CAD build for the part. Positions are in the model's coordinates, mm. A direction names the side the tool comes from. Round coordinates to 2 decimals unless told otherwise and drop trailing zeros. Write each loop counter-clockwise with the first axis right and the second up, starting at its lowest first coordinate (ties: lowest second). Pieces come first, ordered by that corner, then holes. Notation, with made-up numbers: (48.25, 67) - (73.25, 67) arc R38 ccw to (73.25, 105) - close; hole circle Ø8 at (-18.5, 49). An arc over 180 degrees is marked (long way). Use one line per item in the form item = value. Start each with the question number.
Item 1: Pull direction Y, two halves, no side cores. Call faces 4 (the conical face through (-1.429, -3.625, 10.887)), 5 (the flat face through (-1.968, 11, 0)), 6 (the flat face through (0, 6.35, 5)): +Y half, -Y half, draft (parallel to the pull), parting line (faces both ways), or undercut.
Item 2: Tool access for faces 1 (the cylindrical face through (21.804, 3.131, -6.867)), 2 (the flat face through (0, 0, 15)), 3 (the flat face through (1.968, 11, 0)): list every direction of +Z, -Z, +X, -X, +Y, -Y with a clear straight run to the whole face (end or side of a thin tool).
Item 3: Band-saw the part on A-A, the plane y = -183.5. List the corners of the cut face in (x, z) (3 decimals).
Item 4: Pin check, flat tips, straight feed: pin 1 (1 mm diameter, centred on x = -7, y = -152.5, fed in from -Z); pin 2 (5 mm diameter, centred on x = -18, z = 0, fed in from +Y); pin 3 (2.5 mm diameter, centred on y = 10, z = 0.5, fed in from -X). Stop position of each tip, or through.
Item 5: Drill centre lines: L1, parallel to X at y = 4, z = 0; L2, parallel to Z at x = -1, y = -251. Where is each one in solid material? Low to high.
from build123d import *

# Parameters (mm, degrees)
SKETCH1_R                           = 22.86
BOSS_EXTRUDE1_DEPTH                 = 6.35
BOSS_EXTRUDE2_DEPTH                 = 8.89
SKETCH3_R                           = 10.795
BOSS_EXTRUDE3_DEPTH                 = 304.8
CHAMFER1_SIZE                       = 3.81
F_5_32_0_15625_DIAMETER_HOLE1_D     = 3.96875
F_5_32_0_15625_DIAMETER_HOLE1_DEPTH = 6.351
CIRPATTERN1_COUNT                   = 4


with BuildPart() as part:
    # Sketch1 → Boss-Extrude1 (new body)
    with BuildSketch(Plane(origin=(0, 0, 0), x_dir=(1, 0, 0), z_dir=(0, 1, 0))):
        Circle(SKETCH1_R)
    extrude(amount=BOSS_EXTRUDE1_DEPTH)

    # Sketch2 → Boss-Extrude2 (add)
    with BuildSketch(Plane(origin=(0, 6.35, 0), x_dir=(1, 0, 0), z_dir=(0, 1, 0))):
        with BuildLine():
            Line((1.9685, -4.266803107), (1.9685, 4.266803107))
            ThreePointArc((1.9685, 4.266803107), (0, 4.699), (-1.9685, 4.266803107))
            Line((-1.9685, 4.266803107), (-1.9685, -4.266803107))
            ThreePointArc((-1.9685, -4.266803107), (0, -4.699), (1.9685, -4.266803107))
        make_face()
    extrude(amount=BOSS_EXTRUDE2_DEPTH)

    # Sketch3 → Boss-Extrude3 (add)
    with BuildSketch(Plane.XZ):
        Circle(SKETCH3_R)
    extrude(amount=BOSS_EXTRUDE3_DEPTH)

    # Chamfer1
    chamfer1_edges = [part.edges().sort_by_distance(p)[0] for p in [
        (-10.795, 0, 0),
    ]]
    chamfer(chamfer1_edges, length=CHAMFER1_SIZE)

    # 5/32 (0.15625) Diameter Hole1
    with Locations(Plane(origin=(0, 6.35, 0), x_dir=(1, 0, 0), z_dir=(0, 1, 0))):
        with Locations((0, 18)):
            f_5_32_0_15625_diameter_hole1 = Hole(F_5_32_0_15625_DIAMETER_HOLE1_D / 2, depth=F_5_32_0_15625_DIAMETER_HOLE1_DEPTH)

    # CirPattern1: 5/32 (0.15625) Diameter Hole1 ×4 about axis
    cirpattern1_axis = Axis((0, 0, 0), (0, 1, 0))
    for i in range(1, CIRPATTERN1_COUNT):
        add(f_5_32_0_15625_diameter_hole1.rotate(cirpattern1_axis, i * 360 / CIRPATTERN1_COUNT), mode=Mode.SUBTRACT)


solid = part.part
Determined:
q1.face_4 = -Y half
q1.face_5 = draft
q1.face_6 = +Y half
q2.face_1 = +Y, -Y
q2.face_2 = -Y
q2.face_3 = +Z, -Z, +X, +Y
q3.outline = circle Ø21.59 at (0, 0)
q4.pin_1 = -8.62
q4.pin_2 = 6.35
q4.pin_3 = -1.97
q5.L1 = -22.86 to -19.98, -16.02 to 16.02, 19.98 to 22.86
q5.L2 = -10.75 to 10.75
